from build123d import *

# Parameters (mm, degrees)
SKETCH1_R           = 1.9431
BOSS_EXTRUDE1_DEPTH = 2.54
SKETCH2_W           = 38.589880166
SKETCH2_H           = 14.895146316
BOSS_EXTRUDE2_DEPTH = 12.7
CUT_EXTRUDE1_REACH  = 53.659
CUT_EXTRUDE2_DEPTH  = 10
BOSS_EXTRUDE3_DEPTH = 4.7
CUT_EXTRUDE3_DEPTH  = 4.7
CUT_EXTRUDE6_DEPTH  = 51.984917616
BOSS_EXTRUDE4_DEPTH = 20


with BuildPart() as part:
    # Sketch1 → Boss-Extrude1 (new body)
    with BuildSketch(Plane(origin=(0, 0, 0), x_dir=(1, 0, 0), z_dir=(0, 1, 0))):
        with BuildLine():
            Line((-18.7452, 4.565139349), (-2.394218959, 4.565139349))
            ThreePointArc((-2.394218959, 4.565139349), (0.884862389, -0.223028162), (6.223, -2.499694465))
            Line((6.223, -2.499694465), (6.223, -5.842))
            Line((6.223, -5.842), (-12.3952, -39.6494))
            Line((-12.3952, -39.6494), (-18.7452, -39.6494))
            Line((-18.7452, -39.6494), (-18.7452, -5.842))
            Line((-18.7452, -5.842), (-18.7452, 4.565139349))
        make_face()
        with Locations(Location((-15.9512, -28.3464, 0), (0, 0, 270))):
            Circle(SKETCH1_R, mode=Mode.SUBTRACT)
        with Locations(Location((-15.9512, -2.0574, 0), (0, 0, 270))):
            Circle(SKETCH1_R, mode=Mode.SUBTRACT)
    extrude(amount=BOSS_EXTRUDE1_DEPTH)

    # Sketch2 → Boss-Extrude2 (add)
    with BuildSketch(Plane(origin=(7.243438798, 0, 3.989061337), x_dir=(0.48239868494869226, 0, -0.8759517730787308), z_dir=(0.875951773078731, 0, 0.4823986849486923))):
        with Locations((-21.415450328, -4.907573158)):
            Rectangle(SKETCH2_W, SKETCH2_H)
    extrude(amount=BOSS_EXTRUDE2_DEPTH)

    # Cut-Extrude1: up to this face of the body (flat: up to its plane)
    cut_extrude1_end = Plane(part.part.faces().sort_by_distance((2.474947481, -12.355146316, 25.811194672))[0])
    # Sketch3 → Cut-Extrude1 (cut, up to the picked face)
    with BuildSketch(Plane(origin=(0, 2.54, 0), x_dir=(1, 0, 0), z_dir=(0, 1, 0)), mode=Mode.PRIVATE) as cut_extrude1_sk1:
        Polygon((0.318862281, -42.889654691), (2.248457021, -39.385847599), (-8.876130497, -33.2593843), (-10.805725237, -36.763191392), align=None)
    cut_extrude1_tool1 = split(extrude(cut_extrude1_sk1.sketch, amount=-CUT_EXTRUDE1_REACH, mode=Mode.PRIVATE), bisect_by=cut_extrude1_end, keep=Keep.BOTH, mode=Mode.PRIVATE)
    # Sketch3 → Cut-Extrude1 (cut, up to the picked face)
    with BuildSketch(Plane(origin=(0, 2.54, 0), x_dir=(1, 0, 0), z_dir=(0, 1, 0)), mode=Mode.PRIVATE) as cut_extrude1_sk2:
        Polygon((13.82602546, -18.363005045), (15.7556202, -14.859197952), (4.631032681, -8.732734653), (2.701437942, -12.236541746), align=None)
    cut_extrude1_tool2 = split(extrude(cut_extrude1_sk2.sketch, amount=-CUT_EXTRUDE1_REACH, mode=Mode.PRIVATE), bisect_by=cut_extrude1_end, keep=Keep.BOTH, mode=Mode.PRIVATE)
    add(cut_extrude1_tool1.solids().sort_by(Axis((-4.278634, 2.54, 38.074519), (0, -1, 0)))[0], mode=Mode.SUBTRACT)
    add(cut_extrude1_tool2.solids().sort_by(Axis((9.228529, 2.54, 13.54787), (0, -1, 0)))[0], mode=Mode.SUBTRACT)

    # Sketch5 → Cut-Extrude2 (cut)
    with BuildSketch(Plane.XZ.offset(12.355146316)):
        Polygon((-1.270612482, 45.775863299), (17.345094963, 11.972989344), (10.337480778, 8.113799865), (-8.278226667, 41.916673819), align=None)
    extrude(amount=-CUT_EXTRUDE2_DEPTH, mode=Mode.SUBTRACT)

    # Sketch6 → Boss-Extrude3 (add)
    with BuildSketch(Plane(origin=(11.360412132, 0, 6.256335156), x_dir=(0.4823986849486924, 0, -0.8759517730787308), z_dir=(0.8759517730787307, 0, 0.48239868494869237))):
        Polygon((-33.415450328, -2.355146316), (-33.415450328, -12.355146316), (-37.415450328, -12.355146316), (-37.415450328, -2.355146316), (-37.415450328, 2.54), (-33.415450328, 2.54), align=None)
        Polygon((-9.415450328, -12.355146316), (-9.415450328, -2.355146316), (-9.415450328, 2.54), (-5.415450328, 2.54), (-5.415450328, -2.355146316), (-5.415450328, -12.355146316), align=None)
    extrude(amount=-BOSS_EXTRUDE3_DEPTH)

    # Sketch7 → Cut-Extrude3 (cut)
    with BuildSketch(Plane(origin=(11.360412132, 0, 6.256335156), x_dir=(0.4823986849486924, 0, -0.8759517730787308), z_dir=(0.8759517730787307, 0, 0.48239868494869237))):
        Polygon((-21.415450328, -12.355146316), (-33.815450328, -12.355146316), (-33.815450328, -10.755146316), (-37.315450328, -10.755146316), (-37.315450328, -9.055146316), (-33.815450328, -9.055146316), (-33.815450328, -4.601295169), (-9.015450328, -4.601295169), (-9.015450328, -9.055146316), (-5.515450328, -9.055146316), (-5.515450328, -10.755146316), (-9.015450328, -10.755146316), (-9.015450328, -12.355146316), align=None)
    extrude(amount=-CUT_EXTRUDE3_DEPTH, mode=Mode.SUBTRACT)

    # Sketch8 → Cut-Extrude6 (cut, through all)
    with BuildSketch(Plane.XZ):
        with BuildLine():
            Line((-18.7452, 39.6494), (-18.7452, -4.565139349))
            Line((-18.7452, -4.565139349), (-2.394218959, -4.565139349))
            ThreePointArc((-2.394218959, -4.565139349), (0.884862389, 0.223028162), (6.223, 2.499694465))
            Line((6.223, 2.499694465), (6.417585038, 2.467761903))
            Line((6.417585038, 2.467761903), (6.417585038, 5.846526045))
            Line((6.417585038, 5.846526045), (6.220507445, 5.846526045))
            Line((6.220507445, 5.846526045), (-12.3952, 39.6494))
            Line((-12.3952, 39.6494), (-12.3952, 39.814053402))
            Line((-12.3952, 39.814053402), (-18.7452, 39.848024464))
            Line((-18.7452, 39.848024464), (-18.7452, 39.6494))
        make_face()
    extrude(amount=-CUT_EXTRUDE6_DEPTH, mode=Mode.SUBTRACT)

    # Sketch11 → Boss-Extrude4 (add)
    with BuildSketch(Plane(origin=(0, 2.54, 0), x_dir=(1, 0, 0), z_dir=(0, 1, 0))):
        Polygon((6.220507445, -5.846526045), (-12.3952, -39.6494), (-8.50168256, -41.793613586), (10.114024885, -7.990739632), align=None)
    extrude(amount=BOSS_EXTRUDE4_DEPTH)


solid = part.part
Geometry check sheet. Reference: the model listing, model coordinates, mm. A direction names the side the tool comes from. Round coordinates to 2 decimals unless told otherwise and drop trailing zeros. Loops run counter-clockwise (first coordinate to the right, second up) from the corner with the lowest first, then second, coordinate; pieces in that order, holes last.
Item 1: Cross-section at B-B on x = -3. Record the boundary of the cut face in (y, z).
Item 2: Gauge pin test, flat ends, axial feed: pin 1 (13 mm diameter, centred on x = -3, z = 23.5, fed in from -Y); pin 2 (2 mm diameter, centred on x = 10.5, z = 19, fed in from -Y); pin 3 (2 mm diameter, centred on x = 5.5, z = 19.5, fed in from +Y). Record the tip position at first contact, or that the pin passes through.
Item 3: Thickness scan on line 1 (Y direction, x = -1, z = 37); line 2 (Y direction, x = -6.75, z = 31.5); line 3 (X direction, y = 17.5, z = 37). Record the ranges inside material, lowest first.
Item 4: Cross-section at D-D on z = 30. Record the boundary of the cut face in (x, y).
Item 5: Cross-section at C-C on x = -7.25. Record the boundary of the cut face in (y, z), then the cut area to 3 significant figures.
Item 6: Mould release check, pull along Y, two halves, no side actions. Record for faces 4 (the flat face through (-8.67, -9.917, 37.825)), 5 (the flat face through (6.67, -9.89, 9.97)), 6 (the flat face through (-0.487, 0.127, 44.353)), 7 (the flat face through (-1, -4.601, 24)): pulls with the +Y half, pulls with the -Y half, needs draft (parallel to the pull), parting line crosses it, or undercut.
Item 7: Cross-section at A-A on y = -8. Record the boundary of the cut face in (x, z).
Item 8: Access from +Z, -Z, +X, -X, +Y, -Y to the whole of each face (thin tool, end or side, straight path). Record for faces 1 (the flat face through (13, -2.355, 12)), 2 (the flat face through (-1.21, 0.13, 37.48)), 3 (the flat face through (4.982, -6.797, 13.036)).
Answer sheet:
1. outline: (-4.6, 22.59) - (22.54, 22.59) - (22.54, 31.8) - (2.54, 31.8) - (2.54, 36.5) - (-2.36, 36.5) - (-2.36, 32.33) - (-4.6, 32.33) - close; (-2.36, 41.06) - (2.54, 41.06) - (2.54, 44.82) - (-2.36, 44.82) - close
2. pin 1: stops at y = -4.6
2. pin 2: stops at y = -2.36
2. pin 3: stops at y = 2.54
3. line 1: y = -2.36 to 2.54
3. line 2: y = -4.6 to 22.54
3. line 3: x = -10.94 to -5.86
4. outline: (-7.08, -4.6) - (-1.72, -4.6) - (-1.72, -2.36) - (7.42, -2.36) - (7.42, 2.54) - (-2.01, 2.54) - (-2.01, 22.54) - (-7.08, 22.54) - close
5. outline: (-12.36, 34.61) - (-10.76, 34.61) - (-10.76, 38.61) - (-9.06, 38.61) - (-9.06, 34.61) - (-4.6, 34.61) - (-4.6, 30.31) - (22.54, 30.31) - (22.54, 39.52) - (2.54, 39.52) - (2.54, 42.48) - (-2.36, 42.48) - (-2.36, 40.05) - (-12.36, 40.05) - close
5. area: 301 mm2
6. face 4: undercut
6. face 5: undercut
6. face 6: needs draft
6. face 7: pulls with the -Y half
7. outline: (-12.4, 39.65) - (-9.07, 33.61) - (-4.95, 35.88) - (-8.28, 41.92) - close; (2.89, 11.89) - (6.22, 5.85) - (10.34, 8.11) - (7.01, 14.15) - close
8. face 1: +Z, +X, -Y
8. face 2: +Y, -Y
8. face 3: +Z, -X, -Y
